The listing builds one solid part. Answer for the finished solid, in the listing's coordinates (mm). A direction names the side the tool comes from. Coordinates: 2 decimals unless noted, no trailing zeros. Order: outer loops, then holes, each group sorted by start corner. A loop starts at its lowest first (then second) coordinate and runs counter-clockwise, first axis right, second up. Notation, with made-up numbers: (-19.75, 81) -> (19.25, 81) arc R23 cw to (19.25, 97) -> close; hole circle Ø7 at (49.5, 54.25). An arc over 180 degrees is marked (long way). Answer in a Markdown table with one row per item.
```python
from build123d import *

# Parameters (mm, degrees)
SKETCH1_W               = 100
SKETCH1_H               = 26
BOSS_EXTRUDE1_DEPTH     = 2
BOSS_EXTRUDE2_DEPTH     = 100
SKETCH3_W               = 25
SKETCH3_H               = 28
BOSS_EXTRUDE3_DEPTH     = 4
SKETCH4_R               = 2.1
CUT_EXTRUDE1_DEPTH      = 106.39449701
SKETCH5_W               = 120
SKETCH5_H               = 46
SKETCH5_W_2             = 100
SKETCH5_H_2             = 26
CUT_EXTRUDE2_DEPTH      = 105.537074763
CUT_EXTRUDE2_DEPTH_BACK = 105.537074763
SKETCH6_W               = 100
SKETCH6_H               = 26
SKETCH6_R               = 3.6
BOSS_EXTRUDE4_DEPTH     = 4.2
SKETCH8_W               = 100
SKETCH8_H               = 4
BOSS_EXTRUDE5_DEPTH     = 6
SKETCH9_W               = 100
SKETCH9_H               = 4
BOSS_EXTRUDE6_DEPTH     = 10.2
SKETCH10_W              = 4
SKETCH10_H              = 37.5
CUT_EXTRUDE3_DEPTH      = 106.682732743
SKETCH11_W              = 4
SKETCH11_H              = 25
CUT_EXTRUDE4_DEPTH      = 107.737247482
SKETCH13_W              = 10
SKETCH13_H              = 10
BOSS_EXTRUDE7_DEPTH     = 6.2
SKETCH14_W              = 4.2
SKETCH14_H              = 35.5
CUT_EXTRUDE5_DEPTH      = 107.737247482


with BuildPart() as part:
    # Sketch1 → Boss-Extrude1 (new body)
    with BuildSketch(Plane(origin=(0, 0, 0), x_dir=(0, 0, -1), z_dir=(1, 0, 0))):
        with Locations((50, 13)):
            Rectangle(SKETCH1_W, SKETCH1_H)
    extrude(amount=BOSS_EXTRUDE1_DEPTH)

    # Sketch2 → Boss-Extrude2 (add)
    with BuildSketch(Plane.XY):
        Polygon((2, 26), (2, 28), (-12, 28), (-12, 24), (-10, 24), (-10, 26), align=None)
    extrude(amount=-BOSS_EXTRUDE2_DEPTH)

    # Sketch3 → Boss-Extrude3 (add)
    with BuildSketch(Plane(origin=(2, 0, 0), x_dir=(0, 0, -1), z_dir=(1, 0, 0))):
        with Locations((50, 14)):
            Rectangle(SKETCH3_W, SKETCH3_H)
    extrude(amount=BOSS_EXTRUDE3_DEPTH)

    # Sketch4 → Cut-Extrude1 (cut, through all)
    with BuildSketch(Plane(origin=(6, 0, 0), x_dir=(0, 0, -1), z_dir=(1, 0, 0))):
        with Locations((41.5, 21)):
            Circle(SKETCH4_R)
        with Locations((58.5, 21)):
            Circle(SKETCH4_R)
        with Locations((58.5, 4)):
            Circle(SKETCH4_R)
        with Locations((41.5, 4)):
            Circle(SKETCH4_R)
    extrude(amount=-CUT_EXTRUDE1_DEPTH, mode=Mode.SUBTRACT)


with BuildPart() as body_2:
    # Mirror1: mirrored copy
    add(part.part.mirror(Plane(origin=(6, 0, 0), x_dir=(0, 0, 1), z_dir=(1, 0, 0))))

    # Sketch5 → Cut-Extrude2 (cut, two sides)
    with BuildSketch(Plane(origin=(12, 0, 0), x_dir=(0, 0, -1), z_dir=(1, 0, 0))) as cut_extrude2_sk:
        with Locations((50, 13)):
            Rectangle(SKETCH5_W, SKETCH5_H)
        with Locations((50, 13)):
            Rectangle(SKETCH5_W_2, SKETCH5_H_2, mode=Mode.SUBTRACT)
    extrude(amount=CUT_EXTRUDE2_DEPTH, mode=Mode.SUBTRACT)
    extrude(cut_extrude2_sk.sketch, amount=-CUT_EXTRUDE2_DEPTH_BACK, mode=Mode.SUBTRACT)


with BuildPart() as body_2_2:
    # of the pieces the cut leaves, the one that is kept (cut_extrude2_keep)
    add(body_2.part.solids().sort_by_distance((12, 0, 0))[0])

    # Sketch6 → Boss-Extrude4 (add)
    with BuildSketch(Plane(origin=(12, 0, 0), x_dir=(0, 0, -1), z_dir=(1, 0, 0))):
        with Locations((50, 13)):
            Rectangle(SKETCH6_W, SKETCH6_H)
        with Locations((41.5, 21)):
            Circle(SKETCH6_R, mode=Mode.SUBTRACT)
        with Locations((58.5, 21)):
            Circle(SKETCH6_R, mode=Mode.SUBTRACT)
        with Locations((58.5, 4)):
            Circle(SKETCH6_R, mode=Mode.SUBTRACT)
        with Locations((41.5, 4)):
            Circle(SKETCH6_R, mode=Mode.SUBTRACT)
    extrude(amount=BOSS_EXTRUDE4_DEPTH)



with BuildPart() as body_2_3:
    # Sketch8 → Boss-Extrude5 (new body)
    with BuildSketch(Plane(origin=(16.2, 0, 0), x_dir=(0, 0, -1), z_dir=(1, 0, 0))):
        with Locations((50, -2)):
            Rectangle(SKETCH8_W, SKETCH8_H)
    extrude(amount=BOSS_EXTRUDE5_DEPTH)


with BuildPart() as body_2_2_1:
    add(body_2_2.part)

    add(body_2_3.part)  # Boss-Extrude6 merges body 2 3
    # Sketch9 → Boss-Extrude6 (add)
    with BuildSketch(Plane.ZY.offset(-16.2)):
        with Locations((-50, -2)):
            Rectangle(SKETCH9_W, SKETCH9_H)
    extrude(amount=BOSS_EXTRUDE6_DEPTH)

    # Sketch10 → Cut-Extrude3 (cut, through all)
    with BuildSketch(Plane(origin=(0, 0, 0), x_dir=(1, 0, 0), z_dir=(0, 1, 0))):
        with Locations((8, 81.25)):
            Rectangle(SKETCH10_W, SKETCH10_H)
        with Locations((8, 18.75)):
            Rectangle(SKETCH10_W, SKETCH10_H)
    extrude(amount=-CUT_EXTRUDE3_DEPTH, mode=Mode.SUBTRACT)

    # Sketch11 → Cut-Extrude4 (cut, through all)
    with BuildSketch(Plane(origin=(0, 26, 0), x_dir=(1, 0, 0), z_dir=(0, 1, 0))):
        with Locations((8, 50)):
            Rectangle(SKETCH11_W, SKETCH11_H)
    extrude(amount=-CUT_EXTRUDE4_DEPTH, mode=Mode.SUBTRACT)

    # Sketch13 → Boss-Extrude7 (add)
    with BuildSketch(Plane.ZY.offset(-10)):
        with Locations((-50, 31)):
            Rectangle(SKETCH13_W, SKETCH13_H)
    extrude(amount=-BOSS_EXTRUDE7_DEPTH)

    # Sketch14 → Cut-Extrude5 (cut, through all)
    with BuildSketch(Plane(origin=(0, 26, 0), x_dir=(1, 0, 0), z_dir=(0, 1, 0))):
        with Locations((12.1, 17.75)):
            Rectangle(SKETCH14_W, SKETCH14_H)
        with Locations((12.1, 82.25)):
            Rectangle(SKETCH14_W, SKETCH14_H)
    extrude(amount=-CUT_EXTRUDE5_DEPTH, mode=Mode.SUBTRACT)


solid = body_2_2_1.part
```
(1) A cutting plane is placed at D-D, the plane z = -27.5. Determine the outline of the cut face in (x, y).
Check values:
| item | result |
|---|---|
| outline | (14.2, -4) -> (22.2, -4) -> (22.2, 0) -> (16.2, 0) -> (16.2, 26) -> (14.2, 26) -> close |
(2) A cutting plane is placed at A-A, the plane z = -58.5. Determine the outline of the cut face in (x, y).
Check values:
| item | result |
|---|---|
| outline | (10, -4) -> (22.2, -4) -> (22.2, 0) -> (16.2, 0) -> (16.2, 0.4) -> (12, 0.4) -> (12, 1.9) -> (10, 1.9) -> close; (10, 6.1) -> (12, 6.1) -> (12, 7.6) -> (16.2, 7.6) -> (16.2, 17.4) -> (12, 17.4) -> (12, 18.9) -> (10, 18.9) -> close; (10, 23.1) -> (12, 23.1) -> (12, 24.6) -> (16.2, 24.6) -> (16.2, 26) -> (10, 26) -> close |
(3) A cutting plane is placed at B-B, the plane y = 21. Determine the outline of the cut face in (x, z).
Check values:
| item | result |
|---|---|
| outline | (10, -64.5) -> (14.2, -64.5) -> (14.2, -100) -> (16.2, -100) -> (16.2, -62.1) -> (12, -62.1) -> (12, -60.6) -> (10, -60.6) -> close; (10, -56.4) -> (12, -56.4) -> (12, -54.9) -> (16.2, -54.9) -> (16.2, -45.1) -> (12, -45.1) -> (12, -43.6) -> (10, -43.6) -> close; (10, -39.4) -> (12, -39.4) -> (12, -37.9) -> (16.2, -37.9) -> (16.2, 0) -> (14.2, 0) -> (14.2, -35.5) -> (10, -35.5) -> close |
(4) Find the intervals of material crossed by line 1 along Y through (x, z) = (10.65, -41.5); line 2 along Z through (x, y) = (11.1, 4); line 3 along Z through (x, y) = (13.5, 19), in increasing order. Write a range as from..to.
Check values:
| item | result |
|---|---|
| line 1 | -4..1.9, 6.1..18.9, 23.1..26 |
| line 2 | -64.5..-60.6, -56.4..-43.6, -39.4..-35.5 |
| line 3 | -64.5..-61.49, -55.51..-44.49, -38.51..-35.5 |
(5) Which of the six approach directions +Z, -Z, +X, -X, +Y, -Y give full straight-line access (tool end or side, diameter ignored) to faces 4 (the cylindrical face through (14.071, 19.621, -44.825)), 5 (the flat face through (14.4, 26, -72.2)), 6 (the flat face through (14.2, 11, -18)), 7 (the flat face through (14.2, 11, -82)), 8 (the flat face through (16.2, 14, -49))?
Check values:
| item | result |
|---|---|
| face 4 | +X |
| face 5 | -Z, +X, -X, +Y |
| face 6 | +Z, -X, +Y, -Y |
| face 7 | -Z, -X, +Y, -Y |
| face 8 | +Z, -Z, +X, +Y |
(6) Flat-ended cylindrical pins translate along their axes: pin 1 (1 mm diameter, centred on x = 17.5, z = -67.5, fed in from +Y); pin 2 (5 mm diameter, centred on x = 14.5, y = 31, fed in from -Z); pin 3 (6 mm diameter, centred on y = 20.5, z = -57.5, fed in from +X); pin 4 (3 mm diameter, centred on x = 18.5, y = 10.5, fed in from -Z). Find the tip coordinate at first contact, or state that the pin passes through.
Check values:
| item | result |
|---|---|
| pin 1 | y = 0 |
| pin 2 | z = -55 |
| pin 3 | x = 16.2 |
| pin 4 | through |
(7) For a pull along Y with two mould halves and no side action, classify faces 1 (the flat face through (12, 11, -35.5)), 2 (the flat face through (14.4, 26, -27.2)), 3 (the flat face through (12, 19, -60)) as released by +Y, released by -Y, zero draft, split by the parting line, or undercut.
Check values:
| item | result |
|---|---|
| face 1 | zero draft |
| face 2 | released by +Y |
| face 3 | undercut |
(8) A cutting plane is placed at C-C, the plane y = 8.5. Determine the outline of the cut face in (x, z), then the cut area to 3 significant figures.
Check values:
| item | result |
|---|---|
| outline | (10, -64.5) -> (14.2, -64.5) -> (14.2, -100) -> (16.2, -100) -> (16.2, 0) -> (14.2, 0) -> (14.2, -35.5) -> (10, -35.5) -> close |
| area | 322 mm² |
